```python
from build123d import *

# Parameters (mm, degrees)
F0_R     = 0.25
F1_DEPTH = 0.5


# Not quite as in the source:
# - a feature names something its author has since deleted; it is built from what else it names


with BuildPart() as f1:
    # F0 (on Front) → F1 (new body)
    with BuildSketch(Plane.XZ):
        with BuildLine():
            Line((-25.6771374932, 8.2580658644), (-25.1761093938, 8.2580658644))
            Line((-25.1761093938, 8.2580658644), (-25.1761093938, 16.2026529417))
            Line((-25.1761093938, 16.2026529417), (-25.1761093938, 16.2580658644))
            ThreePointArc((-25.1761093938, 16.2580658644), (-25.9255974538, 16.9803594031), (-26.6750855137, 16.2580658644))
            Line((-26.6750855137, 16.2580658644), (-26.6750855137, 16.2026529417))
            Line((-26.6750855137, 16.2026529417), (-26.6750855137, 8.2580658644))
            Line((-26.6750855137, 8.2580658644), (-26.1740574143, 8.2580658644))
            ThreePointArc((-26.1740574143, 8.2580658644), (-25.9255974538, 8.4803594031), (-25.6771374932, 8.2580658644))
        make_face()
        with Locations((-25.9255974538, 16.2303594031)):
            Circle(F0_R, mode=Mode.SUBTRACT)
        with BuildLine():
            ThreePointArc((-26.6750855137, 8.2580658644), (-25.9255974538, 7.4803594031), (-25.1761093938, 8.2580658644))
            Line((-25.1761093938, 8.2580658644), (-25.6771374932, 8.2580658644))
            ThreePointArc((-25.6771374932, 8.2580658644), (-25.6759827606, 8.2442340177), (-25.6755974538, 8.2303594031))
            ThreePointArc((-25.6755974538, 8.2303594031), (-25.9394720684, 7.9807447099), (-26.1740574143, 8.2580658644))
            Line((-26.1740574143, 8.2580658644), (-26.6750855137, 8.2580658644))
        make_face()
    extrude(amount=F1_DEPTH)


solid = f1.part
```
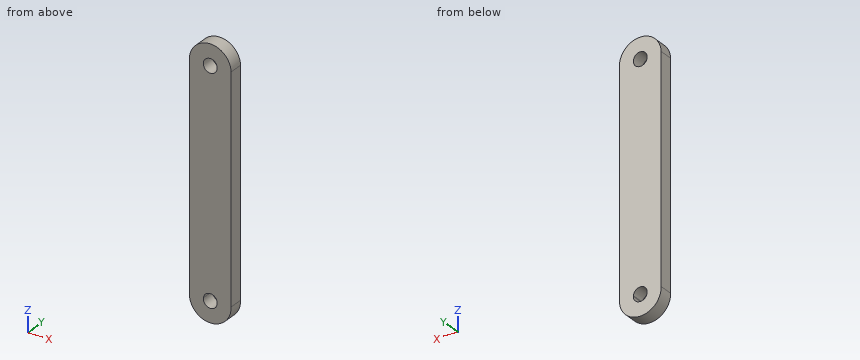
Build history of the part. All positions in model axes, mm. Give positions to 0.01 mm unless a question says otherwise; leave off trailing zeros. Order: outer loops, then holes, each group sorted by start corner. A loop starts at its lowest first (then second) coordinate and runs counter-clockwise, first axis right, second up. Notation, with made-up numbers: M -26,89 L 27,89 A20 ccw 27,119 Z; hole C 35.5,78 d7. An arc over 180 degrees is marked long. Write item = value, one per line. Start each with the question number.
(1) Slice it at C-C on x = -25.35. Write the cut outline in (y, z).
(2) Probe L1, parallel to Z at x = -25.95, y = -0.4; L2, parallel to Z at x = -26.05, y = -0.25; L3, parallel to Z at x = -25.55, y = -0.25. List the from-to ranges inside material, lowest first. Write a range as [from, to].
(3) Slice it at A-A on y = -0.3. Write the cut outline in (x, z).
(4) Slice it at B-B on x = -25.8. Write the cut outline in (y, z).
Responses:
q1.outline = M -0.5,7.75 L 0,7.75 L 0,16.71 L -0.5,16.71 Z
q2.L1 = [7.48, 7.98], [8.48, 15.98], [16.48, 16.98]
q2.L2 = [7.49, 8.01], [8.45, 16.01], [16.45, 16.97]
q2.L3 = [7.58, 16.88]
q3.outline = M -26.68,8.26 A0.75 ccw long -25.18,8.26 L -25.18,16.26 A0.75 ccw -26.68,16.26 Z; hole C -25.93,8.23 d0.5; hole C -25.93,16.23 d0.5
q4.outline = M -0.5,7.49 L 0,7.49 L 0,8.01 L -0.5,8.01 Z; M -0.5,8.45 L 0,8.45 L 0,16.01 L -0.5,16.01 Z; M -0.5,16.45 L 0,16.45 L 0,16.97 L -0.5,16.97 Z
